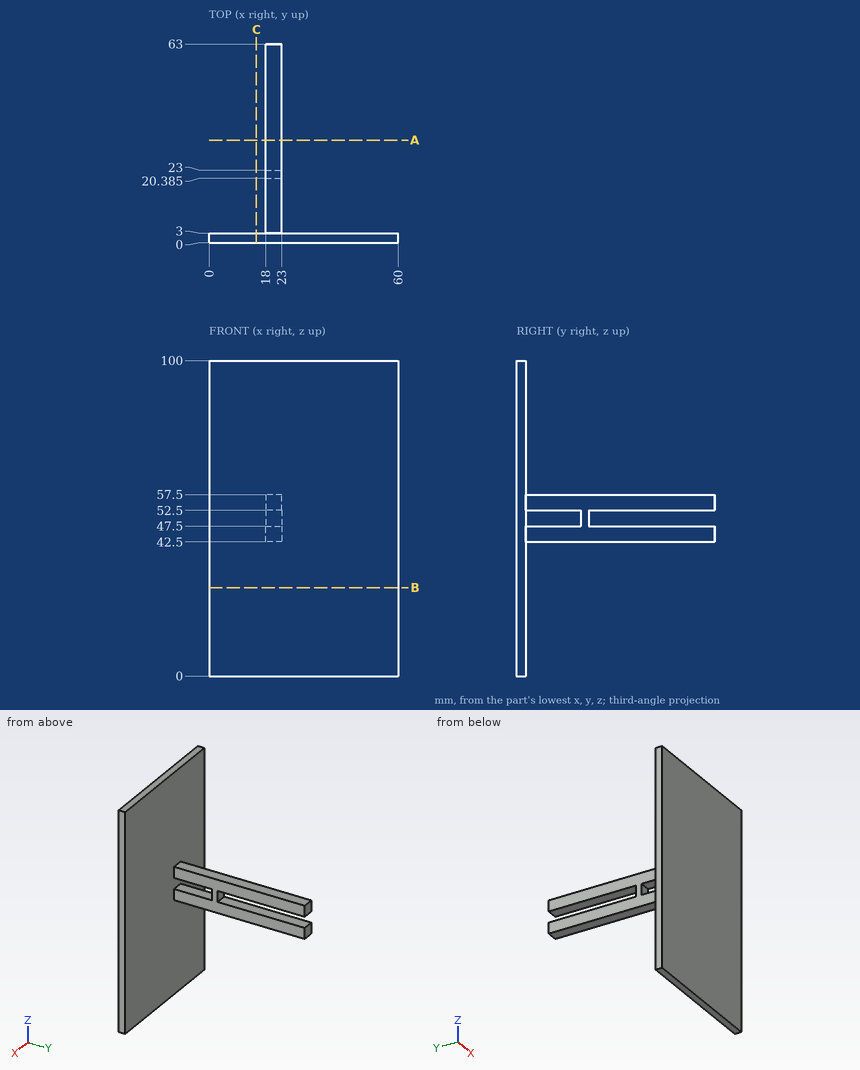
The figure shows three views and two pictorial views of one solid part (mm, origin at its lowest corner). Answer the questions. Give positions to 0.01 mm unless a question says otherwise; leave off trailing zeros. Order: outer loops, then holes, each group sorted by start corner. A loop starts at its lowest first (then second) coordinate and runs counter-clockwise, first axis right, second up. Notation, with made-up numbers: (2.5, 72) -> (24.5, 72) arc R18 cw to (24.5, 98) -> close; hole circle Ø8 at (-11, 81.25). An arc over 180 degrees is marked (long way). One line per item, written item: value.
1) Flat-ended cylindrical pins translate along their axes: P1, Ø4, axis at x = 21.5, y = 10, coming from the -Z side; P2, Ø1.5, axis at x = 21.5, z = 51, coming from the +Y side; P3, Ø16.5, axis at y = 38.5, z = 52.5, coming from the -X side. Find the tip coordinate at first contact, or state that the pin passes through.
Reported:
P1: stops at z = 42.5
P2: stops at y = 23
P3: stops at x = 18
2) Find the intervals of material crossed by line 1 (Z direction, x = 18.5, y = 27); line 2 (Y direction, x = 4.5, z = 18); line 3 (X direction, y = 43, z = 54), in increasing order.
Reported:
line 1: z = 42.5 to 47.5, 52.5 to 57.5
line 2: y = 0 to 3
line 3: x = 18 to 23
3) Find section B-B, the plane z = 28. Determine the outline of the cut face in (x, y), plus the area to 3 significant figures.
Reported:
outline: (0, 0) -> (60, 0) -> (60, 3) -> (0, 3) -> close
area: 180 mm^2
4) Find section C-C, the plane x = 15. Determine the outline of the cut face in (y, z).
Reported:
outline: (0, 0) -> (3, 0) -> (3, 100) -> (0, 100) -> close
5) Find section A-A, the plane y = 32.5. Determine the outline of the cut face in (x, z), plus the area to 3 significant figures.
Reported:
outline: (18, 42.5) -> (23, 42.5) -> (23, 47.5) -> (18, 47.5) -> close; (18, 52.5) -> (23, 52.5) -> (23, 57.5) -> (18, 57.5) -> close
area: 50.0 mm^2
